Autodesk Inventor part; units mm, degrees
ref_plane "YZ Plane" through (0, 0, 0) normal (1, 0, 0) x (0, 1, 0)
ref_plane "XZ Plane" through (0, 0, 0) normal (0, 1, 0) x (-1, 0, 0)
ref_plane "XY Plane" through (0, 0, 0) normal (0, 0, 1) x (1, 0, 0)
sketch "Sketch1" plane through (0, 0, 0) normal (0, 1, 0) x (-1, 0, 0)
  circle A0 centre (0, 0) radius 18
  line L0 (10.3065, -1.0922) -> (4.2236, -9.4646)
  line L1 (2.1462, -10.1396) -> (-7.6962, -6.9416)
  line L2 (-8.9801, -5.1744) -> (-8.9801, 5.1744)
  line L3 (-7.6962, 6.9416) -> (2.1462, 10.1396)
  line L4 (4.2236, 9.4646) -> (10.3065, 1.0922)
  circle A1 centre (3.4301, 10.5567) radius 1.35
  circle A2 centre (11.1, 0) radius 1.35
  circle A3 centre (-8.9801, 6.5244) radius 1.35
  circle A4 centre (-8.9801, -6.5244) radius 1.35
  circle A5 centre (3.4301, -10.5567) radius 1.35
  arc A6 (11.0179, 1.3475) -> (4.6863, 10.0622) centre (0, 0) ccw
  arc A7 (4.6863, -10.0622) -> (11.0179, -1.3475) centre (0, 0) ccw
  arc A8 (-8.1216, -7.5663) -> (2.1232, -10.8951) centre (0, 0) ccw
  arc A9 (2.1232, 10.8951) -> (-8.1216, 7.5663) centre (0, 0) ccw
  arc A10 (-9.7057, 5.386) -> (-9.7057, -5.386) centre (0, 0) ccw
  dimension "d0" = 36
  dimension "d2" = 2.7
  dimension "d3" = 2.7
  dimension "d4" = 2.7
  dimension "d5" = 2.7
  dimension "d6" = 2.7
extrude "Extrusion1" add sketch "Sketch1" along normal blind 5 contours A0 | A2 A7 A5 L0 | L0 A5 L1 A4 L2 A3 L3 A1 L4 A2 | L4 A1 A6 A2 | A5 A8 A4 L1 | L3 A3 A9 A1 | A10 A3 L2 A4
sketch "Sketch2" plane through (0, 5, 0) normal (0, 1, 0) x (1, 0, 0)
  circle A0 centre (0, 0) radius 18
  circle A1 centre (0, 0) radius 15
  point P0 (2.5, -14.7902)
  point P1 (2.5, 14.7902)
  dimension "d9" = 30
extrude "Extrusion2" add sketch "Sketch2" along normal blind 6 contours A1
sketch "Sketch3" plane through (0, 0, 0) normal (0, -1, 0) x (1, 0, 0)
  circle A0 centre (0, 0) radius 18
  line L0 (-8.0829, 0) -> (-4.0415, 7)
  line L1 (-4.0415, 7) -> (4.0415, 7)
  line L2 (4.0415, 7) -> (8.0829, 0)
  line L3 (8.0829, 0) -> (4.0415, -7)
  line L4 (4.0415, -7) -> (-4.0415, -7)
  line L5 (-4.0415, -7) -> (-8.0829, 0)
  dimension "d23" = 14
extrude "Extrusion3" cut sketch "Sketch3" against normal blind 5.5 contours L0 L1 L2 L3 L4 L5
sketch "Sketch4" plane through (0, 5.5, 0) normal (0, -1, 0) x (1, 0, 0)
  circle A0 centre (0, 0) radius 4.5
  dimension "d26" = 9
extrude "Extrusion4" cut sketch "Sketch4" against normal blind 9
chamfer "Chamfer1" distance 3 angle 45 2 edges at (-15, 5, 0) (-15, 11, 0)
equation "\"BendRadius\" = Thickness"
equation "\"BendReliefWidth\" = Thickness"
equation "\"BendReliefDepth\" = 0.5 * Thickness"
equation "\"CornerReliefSize\" = 4 * Thickness"
equation "\"MinimumRemnant\" = 2 * Thickness"
equation "\"TransitionRadius\" = BendRadius"
equation "\"JacobiRadiusSize\" = BendRadius"
equation "\"GapSize\" = Thickness"
properties part number "motorSupportNew1"
Input: part model. Units: mm. Frame: model coordinates. A direction names the side the tool comes from. Round coordinates to 2 decimals unless told otherwise and drop trailing zeros. Loops run counter-clockwise (first coordinate to the right, second up) from the corner with the lowest first, then second, coordinate; pieces in that order, holes last. Notation, with made-up numbers: M -35,79 L 20,79 A34 ccw 20,110 Z; hole C 18,26 d3. An arc over 180 degrees is marked long. Answer in a Markdown table with one row per item. Add a question column.
1. Section B-B (y = 4). Output: boundary loops of the cut face in (x, z).
2. Contact query for flat-ended pins moving along their axis: pin 1 (1.5 mm diameter, centred on x = 9, z = 11, fed in from +Y); pin 2 (0.8 mm diameter, centred on x = -4, z = 11, fed in from -Y); pin 3 (6 mm diameter, centred on x = -5, y = 2, fed in from +Z); pin 4 (3.5 mm diameter, centred on x = -11.1, z = 0, fed in from -Y). Output: stop coordinate, or through.
3. Set-up query: faces 4 (the face through (3.5, 5.5, 3.2)), 5 (the face through (2.343, 2.465, -17.847)). Return all of +Z, -Z, +X, -X, +Y, -Y with unobstructed straight access to the full face (end or side cutting, diameter ignored); none if empty.
4. Mould query, pull axis X, two halves, no side actions, for faces 1 (the face through (-2.64, 10.81, -11.9)), 2 (the face through (6.034, 2.712, 3.549)), 3 (the face through (0, 0, -8)). Classes: released by +X, released by -X, zero draft, split by the parting line, or undercut.
5. Ray query, probe 1 along Y at (x, z) = (4, 6); probe 2 along Y at (x, z) = (-4, -10.5); probe 3 along Z at (x, y) = (0, 8.05). Return the intervals inside material, ascending.
Values follow:
| question | item | result |
|---|---|---|
| 1 | outline | C 0,0 d36; hole C -11.1,0 d2.7; hole M -8.08,0 L -4.04,-7 L 4.04,-7 L 8.08,0 L 4.04,7 L -4.04,7 Z; hole C -3.43,-10.56 d2.7; hole C -3.43,10.56 d2.7; hole C 8.98,-6.52 d2.7; hole C 8.98,6.52 d2.7 |
| 2 | pin 1 | y = 9.54 |
| 2 | pin 2 | y = 5 |
| 2 | pin 3 | z = 17.89 |
| 2 | pin 4 | y = 0 |
| 3 | face 4 | -Y |
| 3 | face 5 | +Y, -Y |
| 4 | face 1 | split by the parting line |
| 4 | face 2 | undercut |
| 4 | face 3 | zero draft |
| 5 | probe 1 | 5.5 to 11 |
| 5 | probe 2 | 5 to 11 |
| 5 | probe 3 | -14.95 to -4.5, 4.5 to 14.95 |
